For this review, take the finished solid that the model builds, in its own axes (mm). A direction names the side the tool comes from. Round coordinates to 2 decimals unless told otherwise and drop trailing zeros. Write each loop counter-clockwise with the first axis right and the second up, starting at its lowest first coordinate (ties: lowest second). Pieces come first, ordered by that corner, then holes.
from build123d import *

# Parameters (mm, degrees)
SKETCH1_W           = 10
SKETCH1_H           = 32
BOSS_EXTRUDE1_DEPTH = 1.4
BOSS_EXTRUDE2_START = -2.9
SKETCH1_3_W         = 10
SKETCH1_3_H         = 32
SKETCH1_3_R         = 2.7
BOSS_EXTRUDE2_DEPTH = 2.9
LPATTERN1_COUNT     = 5
LPATTERN1_PITCH     = 10


with BuildPart() as part:
    # Sketch1 → Boss-Extrude1 (new body)
    with BuildSketch(Plane(origin=(0, 0, 0), x_dir=(1, 0, 0), z_dir=(0, 1, 0))):
        with Locations((5, 16)):
            Rectangle(SKETCH1_W, SKETCH1_H)
        with BuildLine():
            Line((1.00711853, 5.23853211), (2.304805008, 26.961009174))
            ThreePointArc((2.304805008, 26.961009174), (5, 29.5), (7.695194992, 26.961009174))
            Line((7.695194992, 26.961009174), (8.99288147, 5.23853211))
            ThreePointArc((8.99288147, 5.23853211), (8.998219971, 5.119319153), (9, 5))
            ThreePointArc((9, 5), (4.880680847, 1.001780029), (1.00711853, 5.23853211))
        make_face(mode=Mode.SUBTRACT)
    boss_extrude1 = extrude(amount=BOSS_EXTRUDE1_DEPTH)

    # Sketch1_3 → Boss-Extrude2 (add)
    # profile 1 of 3: a face of its own
    with BuildSketch(Plane(origin=(0, 0, 0), x_dir=(1, 0, 0), z_dir=(0, 1, 0)).offset(BOSS_EXTRUDE2_START)):
        with Locations((5, 16)):
            Rectangle(SKETCH1_3_W, SKETCH1_3_H)
        with BuildLine():
            Line((1.00711853, 5.23853211), (2.304805008, 26.961009174))
            ThreePointArc((2.304805008, 26.961009174), (5, 29.5), (7.695194992, 26.961009174))
            Line((7.695194992, 26.961009174), (8.99288147, 5.23853211))
            ThreePointArc((8.99288147, 5.23853211), (8.998219971, 5.119319153), (9, 5))
            ThreePointArc((9, 5), (4.880680847, 1.001780029), (1.00711853, 5.23853211))
        make_face(mode=Mode.SUBTRACT)
    # profile 2 of 3: a face of its own
    with BuildSketch(Plane(origin=(0, 0, 0), x_dir=(1, 0, 0), z_dir=(0, 1, 0)).offset(BOSS_EXTRUDE2_START)):
        with Locations((5, 26.8)):
            Circle(SKETCH1_3_R)
    # profile 3 of 3: a face of its own
    with BuildSketch(Plane(origin=(0, 0, 0), x_dir=(1, 0, 0), z_dir=(0, 1, 0)).offset(BOSS_EXTRUDE2_START)):
        with BuildLine():
            ThreePointArc((7.7, 26.8), (4.919459572, 24.101201519), (2.304805008, 26.961009174))
            Line((2.304805008, 26.961009174), (1.00711853, 5.23853211))
            ThreePointArc((1.00711853, 5.23853211), (5, 9), (8.99288147, 5.23853211))
            Line((8.99288147, 5.23853211), (7.695194992, 26.961009174))
            ThreePointArc((7.695194992, 26.961009174), (7.698798481, 26.880540428), (7.7, 26.8))
        make_face()
    boss_extrude2 = extrude(amount=BOSS_EXTRUDE2_DEPTH)

    # LPattern1: Boss-Extrude1, Boss-Extrude2 ×5
    with Locations(*[(i * LPATTERN1_PITCH, 0, 0) for i in range(1, LPATTERN1_COUNT)]):
        add(boss_extrude1)
        add(boss_extrude2)


solid = part.part
(1) We need section C-C, the plane z = -3.5. Give the boundary of the cut face in (x, y).
Geometry check:
outline: (0, -2.9) - (1.29, -2.9) - (1.29, 1.4) - (0, 1.4) - close; (8.71, -2.9) - (11.29, -2.9) - (11.29, 1.4) - (8.71, 1.4) - close; (18.71, -2.9) - (21.29, -2.9) - (21.29, 1.4) - (18.71, 1.4) - close; (28.71, -2.9) - (31.29, -2.9) - (31.29, 1.4) - (28.71, 1.4) - close; (38.71, -2.9) - (41.29, -2.9) - (41.29, 1.4) - (38.71, 1.4) - close; (48.71, -2.9) - (50, -2.9) - (50, 1.4) - (48.71, 1.4) - close
(2) We need section B-B, the plane y = -2.2. Give the boundary of the cut face in (x, z).
Geometry check:
outline: (0, -32) - (50, -32) - (50, 0) - (0, 0) - close; hole (8.99, -5.24) arc R4 ccw to (9, -5) arc R4 ccw (long way) to start; hole (18.99, -5.24) arc R4 ccw to (19, -5) arc R4 ccw (long way) to start; hole (28.99, -5.24) arc R4 ccw to (29, -5) arc R4 ccw (long way) to start; hole (38.99, -5.24) arc R4 ccw to (39, -5) arc R4 ccw (long way) to start; hole (48.99, -5.24) arc R4 ccw to (49, -5) arc R4 ccw (long way) to start
(3) We need section D-D, the plane y = 0.6. State how many separate pieces and enclosed holes the cut face has, and give its area (3 significant figures).
Geometry check:
separate pieces: 1
enclosed holes: 5
area: 685 mm2
(4) For pin 1 Ø2 at (x, z) = (43, -6.5) entering from -Y; pin 2 Ø2.5 at (x, z) = (15, -21.5) entering from +Y, all flat-tipped, find the tip position at first contact; note any pin that passes through.
Geometry check:
pin 1: passes through
pin 2: stops at y = 0
(5) We need section A-A, the plane x = 5. Give the boundary of the cut face in (y, z).
Geometry check:
outline: (-2.9, -32) - (1.4, -32) - (1.4, -29.5) - (0, -29.5) - (0, -9) - (-2.9, -9) - close; (-2.9, -1) - (1.4, -1) - (1.4, 0) - (-2.9, 0) - close
(6) For line 1 along Z through (x, y) = (35, 0.45); line 2 along X through (y, z) = (-1.6, -1.5); line 3 along X through (y, z) = (0.25, -5.5), list the stretches that pass through material, from the lowest coordinate up.
Geometry check:
line 1: z = -32 to -29.5, -1 to 0
line 2: x = 0 to 3.06, 6.94 to 13.06, 16.94 to 23.06, 26.94 to 33.06, 36.94 to 43.06, 46.94 to 50
line 3: x = 0 to 1.02, 8.98 to 11.02, 18.98 to 21.02, 28.98 to 31.02, 38.98 to 41.02, 48.98 to 50
(7) Mouldability with a two-part tool opening along Z and no side actions: class faces 1 (the face through (25, 0, -18)), 2 (the face through (25, -2.9, -20)), 3 (the face through (25, -1, -32)) as pulls with the +Z half, pulls with the -Z half, needs draft (parallel to the pull), parting line crosses it, or undercut.
Geometry check:
face 1: undercut
face 2: needs draft
face 3: pulls with the -Z half
(8) For faces 4 (the face through (30, 1.4, -20)), 5 (the face through (14.9, 0.7, -29.5)), list the 3-axis set-ups (+Z, -Z, +X, -X, +Y, -Y) from which the entire face can be reached by the end or side of a thin tool; tool diameter is ignored.
Geometry check:
face 4: +Z, -Z, +X, -X, +Y
face 5: +Y
